Build history of the part. All positions in model axes, mm. A direction names the side the tool comes from. Coordinates: 2 decimals unless noted, no trailing zeros. Write each loop counter-clockwise with the first axis right and the second up, starting at its lowest first coordinate (ties: lowest second). Pieces come first, ordered by that corner, then holes.
```python
from build123d import *

# Parameters (mm, degrees)
SKETCH1_W                 = 26.4
SKETCH1_H                 = 26.4
BOSS_EXTRUDE1_DEPTH       = 30
BOSS_EXTRUDE2_DEPTH       = 53
CUT_EXTRUDE1_DEPTH        = 111.157089705
F_6_32_TAPPED_HOLE1_D     = 2.7051
F_1_72_TAPPED_HOLE1_D     = 1.5113
CHAMFER1_SIZE             = 2
M4X0_7_TAPPED_HOLE1_D     = 3.3
M4X0_7_TAPPED_HOLE1_DEPTH = 10.1
M4X0_7_TAPPED_HOLE1_TIP   = 0.991420021
M4X0_7_TAPPED_HOLE2_D     = 3.3
M4X0_7_TAPPED_HOLE2_DEPTH = 10.1
M4X0_7_TAPPED_HOLE2_TIP   = 0.991420021
M4X0_7_TAPPED_HOLE3_D     = 3.3
M4X0_7_TAPPED_HOLE3_DEPTH = 10.1
M4X0_7_TAPPED_HOLE3_TIP   = 0.991420021
CUT_EXTRUDE2_DEPTH        = 111.157089705
M4X0_7_TAPPED_HOLE4_D     = 3.3
M4X0_7_TAPPED_HOLE4_DEPTH = 10.1
M4X0_7_TAPPED_HOLE4_TIP   = 0.991420021
SKETCH24_R                = 5
CUT_EXTRUDE3_DEPTH        = 92.438503925
SKETCH25_W                = 19.328932188
SKETCH25_H                = 1.464466094
SKETCH25_W_2              = 1.464466094
SKETCH25_H_2              = 19.328932188
CUT_EXTRUDE4_DEPTH        = 92.438503925
F_6_32_TAPPED_HOLE2_D     = 2.7051
F_6_32_TAPPED_HOLE2_DEPTH = 15.335533906
F_6_32_TAPPED_HOLE3_D     = 2.7051
F_6_32_TAPPED_HOLE3_DEPTH = 15.335533906
M4X0_7_TAPPED_HOLE6_D     = 3.3
M4X0_7_TAPPED_HOLE6_DEPTH = 10.1
M4X0_7_TAPPED_HOLE6_TIP   = 0.991420021


with BuildPart() as part:
    # Sketch1 → Boss-Extrude1 (new body)
    with BuildSketch(Plane.XY):
        Polygon((-12.426406871, -30), (12.426406871, -30), (30, -12.426406871), (30, 12.426406871), (12.426406871, 30), (-12.426406871, 30), (-30, 12.426406871), (-30, -12.426406871), align=None)
        Rectangle(SKETCH1_W, SKETCH1_H, mode=Mode.SUBTRACT)
    extrude(amount=BOSS_EXTRUDE1_DEPTH)

    # Sketch2 → Boss-Extrude2 (add)
    with BuildSketch(Plane.XY.offset(30)):
        Polygon((14.495689014, 27.930717857), (25.102290732, 17.324116139), (20.859650045, 13.081475452), (10.253048327, 23.68807717), align=None)
        Polygon((-27.930717857, -14.495689014), (-17.324116139, -25.102290732), (-13.081475452, -20.859650045), (-23.68807717, -10.253048327), align=None)
    extrude(amount=BOSS_EXTRUDE2_DEPTH)

    # Sketch3 → Cut-Extrude1 (cut, through all)
    with BuildSketch(Plane(origin=(21.213203436, 21.213203436, 0), x_dir=(0, 0, -1), z_dir=(0.7071067811865475, 0.7071067811865477, 0))):
        Polygon((-83, 9.5), (-83, -5.5), (-68, -5.5), align=None)
    extrude(amount=-CUT_EXTRUDE1_DEPTH, mode=Mode.SUBTRACT)

    # #6-32 Tapped Hole1 (through all)
    with Locations(Plane(origin=(26.736174209, -26.736174209, 37.810660172), x_dir=(0.8660254037844379, 0.2886751345948145, -0.40824829046386363), z_dir=(0.5000000000000013, -0.5000000000000009, 0.7071067811865459))):
        with Locations((-8.826867068, 59.248446925), (-52.917682438, 28.071532389)):
            Hole(F_6_32_TAPPED_HOLE1_D / 2)

    # #1-72 Tapped Hole1 (through all)
    with Locations(Plane(origin=(25.986174209, -25.986174209, 36.75), x_dir=(0.8660254037844379, 0.2886751345948144, -0.40824829046386346), z_dir=(0.5000000000000012, -0.5000000000000009, 0.707106781186546))):
        with Locations((-12.002293548, 63.73917812), (-5.651440587, 54.75771573), (-56.093108918, 32.562263584), (-49.742255957, 23.580801194)):
            Hole(F_1_72_TAPPED_HOLE1_D / 2)

    # Chamfer1
    # the kernel refuses this chamfer: 2 mm, written as the material it takes off along each edge
    with BuildSketch(Plane(origin=(10.253048327, 23.68807717, 30), x_dir=(0.6873969152646597, 0.7262819568766873, 0), z_dir=(0, 0, 1))) as chamfer1_piece_1:
        Polygon((CHAMFER1_SIZE * 0.999621916911, -CHAMFER1_SIZE * 0.0274958766106), (-CHAMFER1_SIZE * 0.0274958766106, -CHAMFER1_SIZE * 0.999621916911), (0, 0), align=None)
    extrude(amount=58.143365976, mode=Mode.SUBTRACT)
    with BuildSketch(Plane(origin=(20.859650045, 13.081475452, 30), x_dir=(-0.7262819568766877, 0.6873969152646593, 0), z_dir=(0, 0, 1)), Plane(origin=(-13.081475452, -20.859650045, 30), x_dir=(-0.6873969152646596, -0.7262819568766873, 0), z_dir=(0, 0, 1))) as chamfer1_piece_2:
        Polygon((CHAMFER1_SIZE * 0.999621916911, -CHAMFER1_SIZE * 0.0274958766106), (-CHAMFER1_SIZE * 0.0274958766106, -CHAMFER1_SIZE * 0.999621916911), (0, 0), align=None)
    extrude(amount=43.143365976, mode=Mode.SUBTRACT)
    with BuildSketch(Plane(origin=(-23.68807717, -10.253048327, 30), x_dir=(-0.7262819568766861, -0.6873969152646611, 0), z_dir=(0, 0, 1))) as chamfer1_piece_3:
        Polygon((CHAMFER1_SIZE * 0.999621916911, CHAMFER1_SIZE * 0.0274958766106), (-CHAMFER1_SIZE * 0.0274958766106, CHAMFER1_SIZE * 0.999621916911), (0, 0), align=None)
    extrude(amount=58.143365976, mode=Mode.SUBTRACT)

    # M4x0.7 Tapped Hole1
    with Locations(Plane.ZY.offset(30)):
        with Locations((7.5, 0), (22.5, 0)):
            Hole(M4X0_7_TAPPED_HOLE1_D / 2, depth=M4X0_7_TAPPED_HOLE1_DEPTH)
            with Locations((0, 0, -(M4X0_7_TAPPED_HOLE1_DEPTH + M4X0_7_TAPPED_HOLE1_TIP / 2))):  # 118° drill point
                Cone(0, M4X0_7_TAPPED_HOLE1_D / 2, M4X0_7_TAPPED_HOLE1_TIP, mode=Mode.SUBTRACT)

    # M4x0.7 Tapped Hole2
    with Locations(Plane(origin=(0, -30, 0), x_dir=(-1, 0, 0), z_dir=(0, -1, 0))):
        with Locations((0, -22.5), (0, -7.5)):
            Hole(M4X0_7_TAPPED_HOLE2_D / 2, depth=M4X0_7_TAPPED_HOLE2_DEPTH)
            with Locations((0, 0, -(M4X0_7_TAPPED_HOLE2_DEPTH + M4X0_7_TAPPED_HOLE2_TIP / 2))):  # 118° drill point
                Cone(0, M4X0_7_TAPPED_HOLE2_D / 2, M4X0_7_TAPPED_HOLE2_TIP, mode=Mode.SUBTRACT)

    # M4x0.7 Tapped Hole3
    with Locations(Plane(origin=(21.213203436, -21.213203436, 0), x_dir=(0, 0, -1), z_dir=(0.7071067811865476, -0.7071067811865475, 0))):
        with Locations((-22.5, 0), (-7.5, 0)):
            Hole(M4X0_7_TAPPED_HOLE3_D / 2, depth=M4X0_7_TAPPED_HOLE3_DEPTH)
            with Locations((0, 0, -(M4X0_7_TAPPED_HOLE3_DEPTH + M4X0_7_TAPPED_HOLE3_TIP / 2))):  # 118° drill point
                Cone(0, M4X0_7_TAPPED_HOLE3_D / 2, M4X0_7_TAPPED_HOLE3_TIP, mode=Mode.SUBTRACT)

    # Sketch20 → Cut-Extrude2 (cut, through all)
    with BuildSketch(Plane(origin=(21.213203436, 21.213203436, 0), x_dir=(0, 0, -1), z_dir=(0.7071067811865475, 0.7071067811865477, 0))):
        Polygon((-83, 9.5), (-81, 9.5), (-81, 7.5), align=None)
    extrude(amount=-CUT_EXTRUDE2_DEPTH, mode=Mode.SUBTRACT)

    # M4x0.7 Tapped Hole4
    with Locations(Plane(origin=(0, 30, 0), x_dir=(1, 0, 0), z_dir=(0, 1, 0))):
        with Locations((0, -7.5), (0, -22.5)):
            Hole(M4X0_7_TAPPED_HOLE4_D / 2, depth=M4X0_7_TAPPED_HOLE4_DEPTH)
            with Locations((0, 0, -(M4X0_7_TAPPED_HOLE4_DEPTH + M4X0_7_TAPPED_HOLE4_TIP / 2))):  # 118° drill point
                Cone(0, M4X0_7_TAPPED_HOLE4_D / 2, M4X0_7_TAPPED_HOLE4_TIP, mode=Mode.SUBTRACT)

    # Sketch24 → Cut-Extrude3 (cut, through all)
    with BuildSketch(Plane(origin=(0, 0, 0), x_dir=(-1, 0, 0), z_dir=(0, 0, -1))):
        with Locations((-9.664466094, 9.664466094)):
            Circle(SKETCH24_R)
        with Locations((9.664466094, 9.664466094)):
            Circle(SKETCH24_R)
        with Locations((9.664466094, -9.664466094)):
            Circle(SKETCH24_R)
        with Locations((-9.664466094, -9.664466094)):
            Circle(SKETCH24_R)
    extrude(amount=-CUT_EXTRUDE3_DEPTH, mode=Mode.SUBTRACT)

    # Sketch25 → Cut-Extrude4 (cut, through all)
    with BuildSketch(Plane(origin=(0, 0, 0), x_dir=(-1, 0, 0), z_dir=(0, 0, -1))):
        with Locations((0, 13.932233047)):
            Rectangle(SKETCH25_W, SKETCH25_H)
        with Locations((-13.932233047, 0)):
            Rectangle(SKETCH25_W_2, SKETCH25_H_2)
    extrude(amount=-CUT_EXTRUDE4_DEPTH, mode=Mode.SUBTRACT)

    # #6-32 Tapped Hole2
    with Locations(Plane(origin=(0, 30, 0), x_dir=(1, 0, 0), z_dir=(0, 1, 0))):
        with Locations((0, -15), (-6.213203436, -7.5), (6.213203436, -7.5), (-6.213203436, -22.5), (6.213203436, -22.5)):
            Hole(F_6_32_TAPPED_HOLE2_D / 2, depth=F_6_32_TAPPED_HOLE2_DEPTH)

    # #6-32 Tapped Hole3
    with Locations(Plane(origin=(30, 0, 0), x_dir=(0, 0, -1), z_dir=(1, 0, 0))):
        with Locations((-15, 0), (-7.5, 6.213203436), (-22.5, -6.213203436), (-22.5, 6.213203436), (-7.5, -6.213203436)):
            Hole(F_6_32_TAPPED_HOLE3_D / 2, depth=F_6_32_TAPPED_HOLE3_DEPTH)

    # M4x0.7 Tapped Hole6
    with Locations(Plane(origin=(30, 0, 0), x_dir=(0, 0, -1), z_dir=(1, 0, 0))):
        with Locations((-22.5, 0), (-7.5, 0)):
            Hole(M4X0_7_TAPPED_HOLE6_D / 2, depth=M4X0_7_TAPPED_HOLE6_DEPTH)
            with Locations((0, 0, -(M4X0_7_TAPPED_HOLE6_DEPTH + M4X0_7_TAPPED_HOLE6_TIP / 2))):  # 118° drill point
                Cone(0, M4X0_7_TAPPED_HOLE6_D / 2, M4X0_7_TAPPED_HOLE6_TIP, mode=Mode.SUBTRACT)


solid = part.part
```
1. Flat gauge pins, fed straight in: pin 1 (2 mm diameter, centred on x = 18.5, y = 16.5, fed in from +Z); pin 2 (3 mm diameter, centred on x = -23.5, z = 61.5, fed in from +Y); pin 3 (3 mm diameter, centred on x = -19, z = 44.5, fed in from +Y); pin 4 (1.5 mm diameter, centred on y = 12, z = 62, fed in from +X). Where does each tip first touch, or does it go through?
Computed values:
pin 1: stops at z = 73.09
pin 2: stops at y = -11.67
pin 3: stops at y = -13.44
pin 4: passes through
2. Probe line 1 along Z through (x, y) = (0, -22.75); line 2 along Y through (x, z) = (19.5, 23); line 3 along X through (y, z) = (-4, 18.5). List the from-to ranges inside material, lowest first.
Computed values:
line 1: z = 0 to 5.85, 9.15 to 20.85, 24.15 to 30
line 2: y = -22.93 to -21.72, -17.28 to -7.47, -4.96 to -0.85, 0.85 to 4.96, 7.47 to 22.93
line 3: x = -30 to -13.2, 14.66 to 30
3. Mould opens along Y. For faces 1 (the face through (21.09, -21.336, 14.79)), 2 (the face through (-3, 30, 15)), 3 (the face through (14.683, 23.818, 75.919)), 4 (the face through (-6.94, 22.22, 21.36)) say: +Y half, -Y half, draft (parallel to the pull), parting line (faces both ways), or undercut.
Computed values:
face 1: -Y half
face 2: +Y half
face 3: undercut
face 4: draft
4. 3-axis set-ups, long thin cutter, end or side, ignore diameter. For faces 5 (the face through (0.215, 24.879, 20.864)), 6 (the face through (-14.496, -21, 50)), 7 (the face through (22.22, -6.73, 23.75)): which of +Z, -Z, +X, -X, +Y, -Y reach the whole face in a straight line?
Computed values:
face 5: +Y
face 6: +Z, +X, +Y, -Y
face 7: +X
5. Saw through at A-A on z = 19.5. List the corners of the cut face in (x, y), plus the area to 3 significant figures.
Computed values:
outline: (-30, -12.43) - (-12.43, -30) - (12.43, -30) - (30, -12.43) - (30, 12.43) - (12.43, 30) - (-12.43, 30) - (-30, 12.43) - close; hole (-13.2, -6.13) arc R5 ccw to (-6.13, -13.2) - (6.13, -13.2) arc R5 ccw to (14.66, -9.66) - (14.66, 9.66) arc R5 ccw to (9.66, 14.66) - (-9.66, 14.66) arc R5 ccw to (-13.2, 6.13) - close
area: 2,190 mm2
